Autodesk Inventor part; units mm, degrees
ref_plane "YZ Plane" through (0, 0, 0) normal (1, 0, 0) x (0, 1, 0)
ref_plane "XZ Plane" through (0, 0, 0) normal (0, 1, 0) x (-1, 0, 0)
ref_plane "XY Plane" through (0, 0, 0) normal (0, 0, 1) x (1, 0, 0)
sketch "Esboço1" plane through (0, 0, 0) normal (0, 1, 0) x (-1, 0, 0)
  line L0 (0, 0) -> (0, -190)
  line L1 (0, -190) -> (150, -190)
  line L2 (150, -190) -> (150, 0)
  line L3 (150, 0) -> (0, 0)
  dimension "d0" = 190
  dimension "d1" = 150
extrude "Extrusão1" add sketch "Esboço1" along normal mid plane 5
fillet "Arredondamento1" radius 40 1 edges at (0, 0, 0)
fillet "Arredondamento2" radius 40 3 edges at (-150, 0, 0) (0, 0, -190) (-150, 0, -190)
sketch "Esboço2" plane through (0, 2.5, 0) normal (0, 1, 0) x (1, 0, 0)
  line L0 (-110, 0) -> (-40, 0)
  line L1 (-150, 150) -> (-150, 40)
  line L2 (0, 40) -> (0, 150)
  line L3 (0, 110) -> (5, 110)
  line L4 (-150, 110) -> (-155, 110)
  line L5 (-155, 110) -> (-155, 175)
  line L6 (-155, 175) -> (-150, 175)
  line L7 (0, 175) -> (5, 175)
  line L8 (5, 175) -> (5, 110)
  line L9 (-155, 175) -> (-155, 180)
  line L10 (-155, 180) -> (-115.1221, 180)
  line L11 (-155, 110) -> (-155, 105)
  line L12 (-155, 105) -> (-150, 105)
  line L13 (5, 110) -> (5, 105)
  line L14 (5, 105) -> (0, 105)
  line L15 (-115.1221, 180) -> (-136.4575, 180)
  arc A0 (-110, 190) -> (-150, 150) centre (-110, 150) ccw
  line L16 (5, 175) -> (5, 180)
  line L17 (5, 180) -> (11.9999, 180)
  line L18 (-150, 175) -> (-141.225, 175)
  line L19 (0, 175) -> (-8.775, 175)
  arc A1 (0, 150) -> (-40, 190) centre (-40, 150) ccw
  line L20 (11.9999, 180) -> (-13.5425, 180)
  line L21 (0, 150) -> (0, 175)
  arc A2 (-110, 190) -> (-150, 150) centre (-110, 150) ccw
  line L22 (-150, 150) -> (-150, 175)
  point P0 (0, 0)
  point P1 (-136.4575, 180)
  dimension "d162" = 5
  dimension "d163" = 5
  dimension "d165" = 5
  dimension "d166" = 5
sketch "Esboço5" plane through (0, 2.5, 0) normal (0, 1, 0) x (1, 0, 0)
  circle A0 centre (-120.0001, 23.5) radius 2.5
  circle A1 centre (-30.5501, 23.5) radius 2.5
  circle A2 centre (-92.8994, 163.5564) radius 2.5
  circle A3 centre (-56.8994, 163.5564) radius 2.5
  point P0 (0, 0)
  dimension "d69" = 5
  dimension "d70" = 5
  dimension "d116" = 5
  dimension "d117" = 5
extrude "Extrusão17" cut sketch "Esboço5" against normal through all
extrude "Extrusão20" add sketch "Esboço2" against normal blind 5 contours L22 L18 A0 | L1 L12 L11 L4 | L18 L6 L9 L10 A0 | L2 L3 L13 L14 | A1 L19 L21 | A1 L20 L16 L7 L19
sketch "Esboço7" plane through (0, 2.5, 0) normal (0, 1, 0) x (1, 0, 0)
  line L0 (-150, 110) -> (-150, 175)
  line L1 (-126.8835, 155.0003) -> (-150, 155.0003)
  line L2 (-28.2595, 155.0003) -> (0, 155.0003)
  line L3 (-126.8835, 130.0003) -> (-150, 130.0003)
  line L4 (-126.8835, 130.0003) -> (-90, 130.0003)
  line L5 (-90, 130.0003) -> (-90, 155.0003)
  line L6 (-90, 155.0003) -> (-126.8835, 155.0003)
  line L7 (-28.2595, 130.0003) -> (0, 130.0003)
  line L8 (0, 175) -> (0, 110)
  line L9 (-28.2595, 130.0003) -> (-60, 130.0003)
  line L10 (-60, 130.0003) -> (-60, 155.0003)
  line L11 (-60, 155.0003) -> (-28.2595, 155.0003)
  line L12 (0, 155.0003) -> (0, 130.0003)
  line L13 (-150, 155.0003) -> (-150, 130.0003)
  point P0 (0, 0)
  point P1 (0, 142.5003)
  point P2 (-150, 142.5)
  point P3 (-90, 142.5003)
  dimension "d170" = 25
  dimension "d216" = 60
  dimension "d252" = 60
sketch "Esboço8" plane through (0, 2.5, 0) normal (0, 1, 0) x (1, 0, 0)
  line L0 (0, 175) -> (0, 110)
  circle A0 centre (-5, 125.0003) radius 2.5
  line L1 (-150, 155.0003) -> (-84.9995, 155.0003)
  circle A1 centre (-145.0006, 160.0003) radius 2.5
  circle A2 centre (-145, 125.0003) radius 2.5
  circle A3 centre (-5, 160.0003) radius 2.5
  point P0 (0, 0)
  point P1 (0, 130.0003)
  dimension "d180" = 5
  dimension "d186" = 5
  dimension "d187" = 5
  dimension "d264" = 5
extrude "Extrusão30" cut sketch "Esboço7" against normal through all
extrude "Extrusão32" cut sketch "Esboço8" against normal through all
sketch "Esboço10" plane through (0, 2.5, 0) normal (0, 1, 0) x (1, 0, 0)
  line L0 (5, 180) -> (-13.5425, 180)
  line L1 (0, 180) -> (0, 104.8979)
  line L2 (0, 104.8979) -> (5, 104.8979)
  line L3 (5, 104.8979) -> (5, 180)
  line L4 (5, 180) -> (0, 180)
  line L5 (-150, 175) -> (-150, 155.0003)
  line L6 (-150, 175) -> (-150, 180)
  line L7 (-136.4575, 180) -> (-155, 180)
  line L8 (-150, 180) -> (-155, 180)
  line L9 (-155, 180) -> (-155, 104.8979)
  line L10 (-155, 104.8979) -> (-150, 104.8979)
  line L11 (-150, 175) -> (-150, 104.8979)
  point P0 (0, 0)
extrude "Extrusão33" cut sketch "Esboço10" against normal through all
sketch "Esboço6" plane through (0, 2.5, 0) normal (0, 1, 0) x (1, 0, 0)
  line L0 (-40, 0) -> (-110, 0)
  line L1 (-75, 0) -> (-57.5, 0)
  line L2 (-92.5, 45) -> (-92.5, 0)
  line L3 (-75, 0) -> (-92.5, 0)
  line L4 (-92.5, 45) -> (-57.5, 45)
  circle A0 centre (-69.65, 48.6) radius 2.5
  line L5 (-75, 45) -> (-86, 45)
  line L6 (-86, 45) -> (-86, 57)
  line L7 (-86, 57) -> (-64, 57)
  line L8 (-64, 57) -> (-64, 45)
  line L9 (-60, 39) -> (-90, 39)
  line L10 (-60, 15) -> (-90, 15)
  circle A1 centre (-90, 39) radius 2.5
  circle A2 centre (-60, 39) radius 2.5
  circle A3 centre (-60, 15) radius 2.5
  circle A4 centre (-90, 15) radius 2.5
  point P0 (0, 0)
  dimension "d137" = 45
  dimension "d138" = 35
  dimension "d159" = 5
  dimension "d206" = 11
  dimension "d207" = 12
  dimension "d208" = 22
  dimension "d349" = 5
  dimension "d350" = 5
  dimension "d351" = 5
  dimension "d352" = 5
sketch "Esboço11" plane through (0, 2.5, 0) normal (0, 1, 0) x (1, 0, 0)
  line L0 (-150, 130.0003) -> (-150, 40)
  circle A0 centre (-146.5001, 117.8649) radius 1.375
  circle A1 centre (-88.5001, 117.8649) radius 1.375
  circle A2 centre (-88.5001, 68.8649) radius 1.375
  circle A3 centre (-146.5001, 68.8649) radius 1.375
  point P0 (0, 0)
  dimension "d292" = 2.75
  dimension "d293" = 2.75
  dimension "d294" = 2.75
  dimension "d295" = 2.75
extrude "Extrusão35" cut sketch "Esboço11" against normal through all
extrude "Extrusão39" cut sketch "Esboço6" against normal through all contours A2 | A1 | A3 | A4
sketch "Esboço13" plane through (0, 2.5, 0) normal (0, 1, 0) x (1, 0, 0)
  circle A0 centre (-142.1978, 23.0054) radius 1.5
  arc A1 (-150, 40) -> (-110, 0) centre (-110, 40) ccw
  circle A2 centre (-126.995, 7.8026) radius 1.5
  line L0 (-146.2103, 23.0054) -> (-126.995, 3.7899)
  line L1 (-146.2103, 23.0054) -> (-146.2103, 3.7899)
  line L2 (-146.2103, 3.7899) -> (-126.995, 3.7899)
  circle A3 centre (-7.8022, 23.0054) radius 1.5
  arc A4 (-40, 0) -> (0, 40) centre (-40, 40) ccw
  circle A5 centre (-23.005, 7.8026) radius 1.5
  line L3 (-3.7897, 23.0054) -> (-23.005, 3.7899)
  line L4 (-3.7897, 23.0054) -> (-3.7897, 3.7899)
  line L5 (-3.7897, 3.7899) -> (-23.005, 3.7899)
  point P0 (0, 0)
extrude "Extrusão41" cut sketch "Esboço13" against normal through all contours L0 A1 | A1 L2 L1 | L3 A4 | A4 L4 L5
sketch "Esboço12" plane through (0, 2.5, 0) normal (0, 1, 0) x (1, 0, 0)
  line L0 (-40, 0) -> (-110, 0)
  line L1 (-53.5, 10) -> (-53.5, 17)
  line L2 (-53.5, 17) -> (-96.5, 17)
  line L3 (-96.5, 17) -> (-96.5, 10)
  arc A0 (-40, 0) -> (0, 40) centre (-40, 40) ccw
  arc A1 (-150, 40) -> (-110, 0) centre (-110, 40) ccw
  line L4 (-110, 0) -> (-150, 40)
  line L5 (-150, 40) -> (-145.0503, 44.9497)
  line L6 (-145.0503, 44.9497) -> (-105.0503, 4.9497)
  line L7 (-40, 0) -> (0, 40)
  line L8 (0, 40) -> (-4.9497, 44.9497)
  line L9 (-4.9497, 44.9497) -> (-44.9497, 4.9497)
  line L10 (-44.9497, 4.9497) -> (-40, 0)
  line L11 (-110, 0) -> (-105.0503, 4.9497)
  line L12 (-112.3225, 2.3225) -> (-109.1405, 5.5045)
  circle A2 centre (-85.75, 4.5) radius 1.5
  circle A3 centre (-75, 4.5) radius 1.5
  circle A4 centre (-64.25, 4.5) radius 1.5
  line L13 (-134.4196, 30.7835) -> (-137.6016, 27.6016)
  line L14 (-126.8182, 23.1821) -> (-130, 20)
  line L15 (-119.2168, 15.5807) -> (-122.3988, 12.3988)
  line L16 (-30.7832, 15.5807) -> (-27.6012, 12.3988)
  line L17 (-23.1818, 23.1821) -> (-19.9998, 20.0002)
  line L18 (-15.5804, 30.7835) -> (-12.3984, 27.6016)
  line L19 (-146.2103, 23.0054) -> (-126.995, 3.7899)
  circle A5 centre (-125.819, 8.9785) radius 1.5
  circle A6 centre (-133.4203, 16.5797) radius 1.5
  circle A7 centre (-141.0218, 24.1813) radius 1.5
  line L20 (-3.7897, 23.0054) -> (-23.005, 3.7899)
  circle A8 centre (-24.181, 8.9785) radius 1.5
  circle A9 centre (-16.5796, 16.5799) radius 1.5
  circle A10 centre (-8.9782, 24.1813) radius 1.5
  point P0 (0, 0)
  dimension "d301" = 7
  dimension "d310" = 7
  dimension "d311" = 7
  dimension "d325" = 4.5
  dimension "d356" = 3
  dimension "d357" = 3
  dimension "d358" = 3
  dimension "d374" = 3
  dimension "d375" = 3
  dimension "d376" = 3
  dimension "d379" = 3
  dimension "d380" = 3
  dimension "d381" = 3
extrude "Extrusão42" cut sketch "Esboço12" against normal through all contours A2 | A3 | A4 | A5 | A6 | A7 | A8 | A9 | A10
sketch "Esboço14" plane through (0, 2.5, 0) normal (0, 1, 0) x (1, 0, 0)
  line L0 (-63.9015, 51) -> (-63.9015, 45.1)
  line L1 (-63.9015, 51) -> (-63.9015, 56.9)
  line L2 (-63.9015, 56.9) -> (-86.1015, 56.9)
  line L3 (-86.1015, 56.9) -> (-86.1015, 51)
  line L4 (-86.1015, 51) -> (-86.1015, 45.1)
  line L5 (-86.1015, 45.1) -> (-63.9015, 45.1)
  circle A0 centre (-59.9015, 51) radius 1
  circle A1 centre (-90.1015, 51) radius 1
  point P0 (0, 0)
  point P1 (-60.9815, 51)
  dimension "d384" = 2.92
  dimension "d385" = 22.2
  dimension "d386" = 5.9
  dimension "d387" = 5.9
  dimension "d392" = 2
  dimension "d393" = 2
extrude "Extrusão43" cut sketch "Esboço14" against normal through all
properties part number "BaseP"
Work out the finished part from the listing and answer in its coordinate system (mm). A direction names the side the tool comes from. Coordinates: 2 decimals unless noted, no trailing zeros. Write each loop counter-clockwise with the first axis right and the second up, starting at its lowest first coordinate (ties: lowest second). Pieces come first, ordered by that corner, then holes. Notation, with made-up numbers: M -38.5,80.5 L -24.5,80.5 A26 ccw -24.5,112.5 Z; hole C 64.25,62 d1. An arc over 180 degrees is marked long. Write item = value, one per line.
1. Determine the mould class of faces 4 (the face through (0, 0, -168)), 5 (the face through (-142.69, 0.04, -124.04)), 6 (the face through (-149.014, -0.035, -31.174)), 7 (the face through (-143, 0, -180)) for opening direction Z: released by +Z, released by -Z, zero draft, split by the parting line, or undercut.
Solution:
face_4 = zero draft
face_5 = undercut
face_6 = released by +Z
face_7 = released by -Z
2. The part is cut by section B-B (y = 0.95). State how many separate pieces and enclosed holes the cut face has, then the cut area to 3 significant figures.
Solution:
separate_pieces = 1
enclosed_holes = 28
area = 23,700 mm2
3. For faces 1 (the face through (-136.737, 0.035, -13.532)), 2 (the face through (-86.102, 0, -51)), 3 (the face through (-30, 0, -130)), determine the directions among +Z, -Z, +X, -X, +Y, -Y from which every point of the face is accessible in a straight line to the end or side of a thin tool.
Solution:
face_1 = +Z, -X, +Y, -Y
face_2 = +Y, -Y
face_3 = +X, +Y, -Y
4. Straight lines are drawn through the part: line 1 (Z direction, x = -64, y = -1.45); line 2 (Z direction, x = -66.5, y = -1.6); line 3 (Z direction, x = -45.5, y = -0.95). For each, find the intervals that lie inside material, in ascending order. Write a range as from..to.
Solution:
line_1 = -190..-56.9, -45.1..-5.98, -3.02..0
line_2 = -190..-56.9, -45.1..0
line_3 = -190..-155, -130..0
5. Flat-ended cylindrical pins translate along their axes: pin 1 (6 mm diameter, centred on x = -5, z = -125, fed in from -Y); pin 2 (1.5 mm diameter, centred on x = -30.5, y = -1.5, fed in from -Z); pin 3 (2.5 mm diameter, centred on y = 0, z = -143, fed in from +X). Find the tip coordinate at first contact, or state that the pin passes through.
Solution:
pin_1 = -2.5
pin_2 = -189.03
pin_3 = -60
6. The part is cut by section A-A (x = -104). Determine the outline of the cut face in (y, z).
Solution:
outline = M -2.5,-190 L 2.5,-190 L 2.5,-155 L -2.5,-155 Z; M -2.5,-130 L 2.5,-130 L 2.5,0 L -2.5,0 Z
